Drawing for the job (mm, zero at the part's lowest x, y, z). Coordinates: 2 decimals unless noted, no trailing zeros. Order: outer loops, then holes, each group sorted by start corner. A loop starts at its lowest first (then second) coordinate and runs counter-clockwise, first axis right, second up.
1) Wall check: L1, parallel to Z at x = 8, y = 4.75; L2, parallel to X at y = 4.5, z = 45.5; L3, parallel to X at y = 3, z = 87.5. Give the ranges that are in metal, low to high.
2) Cut at B-B (z = 111). List the corners of the cut face in (x, y), and give its area (3 significant figures).
3) Cut at A-A (x = 4). List the corners of the cut face in (y, z).
4) Pin check, flat tips, straight feed: pin 1 Ø1.5 at (y, z) = (1.5, 42) entering from +X (1 decimal); pin 2 Ø4 at (y, z) = (5, 60.5) entering from -X; pin 3 Ø2 at (x, y) = (2.5, 4) entering from -Z. Stop position of each tip, or through.
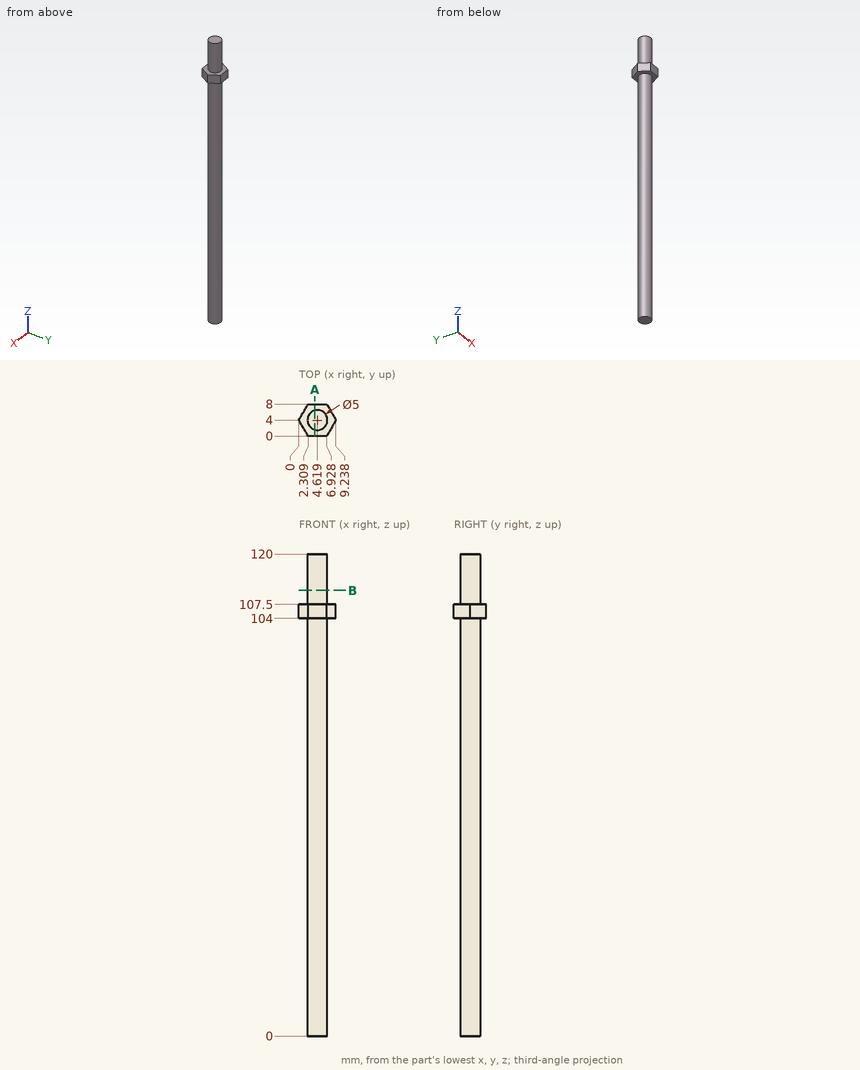
Geometry check:
1. L1: z = 104 to 107.5
1. L2: x = 2.17 to 7.07
1. L3: x = 2.33 to 6.91
2. outline: circle Ø5 at (4.62, 4)
2. area: 19.6 mm2
3. outline: (0, 104) - (1.58, 104) - (1.58, 0) - (6.42, 0) - (6.42, 104) - (8, 104) - (8, 107.5) - (6.42, 107.5) - (6.42, 120) - (1.58, 120) - (1.58, 107.5) - (0, 107.5) - close
4. pin 1: stops at x = 6.4
4. pin 2: stops at x = 2.12
4. pin 3: stops at z = 0
